Part model, mm, in its own coordinate system. A direction names the side the tool comes from. Round coordinates to 2 decimals unless told otherwise and drop trailing zeros. Write each loop counter-clockwise with the first axis right and the second up, starting at its lowest first coordinate (ties: lowest second). Pieces come first, ordered by that corner, then holes. Notation, with made-up numbers: M 18.5,31 L 42.5,31 A10 ccw 42.5,50 Z; hole C -17,41.5 d9. An arc over 180 degrees is marked long. One line per question, with ' | ' between items. Start each with the question number.
1) Saw through at C-C (x = -12.7). List the corners of the cut face in (y, z), plus the area to 3 significant figures.
2) Saw through at B-B (y = 25.4). List the corners of the cut face in (x, z), plus the area to 3 significant figures.
3) Tool access for faces 4 (the face through (-25.4, 113, 13)), 5 (the face through (-72, 239, 23.812)), 6 (the face through (-130, 252.412, 13)): list every direction of +Z, -Z, +X, -X, +Y, -Y with a clear straight run to the whole face (end or side of a thin tool).
4) Wall check: probe 1 along Y at (x, z) = (-73, 13); probe 2 along X at (y, z) = (34, 16); probe 3 along Y at (x, z) = (-12.7, 0.9). Give the ranges that are in metal, low to high. Write a range as [from, to].
5) Drop flat-ended pins along their axis: pin 1 Ø12 at (x, z) = (-178, 11.5) entering from -Y; pin 2 Ø8 at (y, z) = (185, 3.5) entering from -X. Give the stop position or say it passes through.
6) Saw through at D-D (y = 241.3). List the corners of the cut face in (x, z), plus the area to 3 significant figures.
7) Saw through at A-A (z = 9.75). List the corners of the cut face in (x, y), plus the area to 3 significant figures.
8) Mould opens along X. For faces 1 (the face through (-249.018, 242.731, 0.783)), 2 (the face through (-137, 230.188, 13)), 3 (the face through (0, 129, 13)) say: pulls with the +X half, pulls with the -X half, needs draft (parallel to the pull), parting line crosses it, or undercut.
Autodesk Inventor part; units mm, degrees
ref_plane "YZ Plane" through (0, 0, 0) normal (1, 0, 0) x (0, 1, 0)
ref_plane "XZ Plane" through (0, 0, 0) normal (0, 1, 0) x (-1, 0, 0)
ref_plane "XY Plane" through (0, 0, 0) normal (0, 0, 1) x (1, 0, 0)
sketch "Sketch1" plane through (0, 0, 0) normal (0, 0, 1) x (1, 0, 0)
  line L0 (0, 0) -> (-25.4, 0)
  line L1 (-254, 228.6) -> (-254, 254)
  line L2 (-254, 254) -> (0, 254)
  line L3 (0, 254) -> (0, 0)
  line L4 (-25.4, 0) -> (-25.4, 228.6)
  line L5 (-25.4, 228.6) -> (-254, 228.6)
  dimension "d0" = 25.4
  dimension "d1" = 254
  dimension "d2" = 254
extrude "Extrusion1" add sketch "Sketch1" along normal blind 25.4
shell "Shell1" thickness 1.5875 removed faces 2 at (-8.4667, 0, 8.4667) at (-254, 237.0667, 8.4667)
sketch "Sketch2" plane through (0, 0, 25.4) normal (0, 0, 1) x (1, 0, 0)
  line L0 (0, 0) -> (-25.4, 0)
  line L1 (0, 254) -> (0, 0)
  circle A0 centre (-12.7, 25.4) radius 4.7625
  dimension "d6" = 9.525
  dimension "d7" = 12.7
  dimension "d8" = 25.4
extrude "Extrusion2" cut sketch "Sketch2" against normal through all
sketch "Sketch3" plane through (0, 0, 0) normal (0, 0, -1) x (-1, 0, 0)
  line L0 (25.4, 228.6) -> (254, 228.6)
  line L1 (254, 228.6) -> (254, 254)
  circle A0 centre (244.475, 241.3) radius 4.7625
  dimension "d11" = 9.525
  dimension "d12" = 12.7
  dimension "d13" = 9.525
extrude "Extrusion3" cut sketch "Sketch3" against normal through all
properties part number "LoweringArm" material "Aluminum-6061"
Answer key:
1) outline: M 0,0 L 20.64,0 L 20.64,1.59 L 0,1.59 Z; M 0,23.81 L 20.64,23.81 L 20.64,25.4 L 0,25.4 Z; M 30.16,0 L 254,0 L 254,25.4 L 30.16,25.4 L 30.16,23.81 L 252.41,23.81 L 252.41,1.59 L 30.16,1.59 Z | area: 811 mm2
2) outline: M -25.4,0 L -17.46,0 L -17.46,1.59 L -23.81,1.59 L -23.81,23.81 L -17.46,23.81 L -17.46,25.4 L -25.4,25.4 Z; M -7.94,0 L 0,0 L 0,25.4 L -7.94,25.4 L -7.94,23.81 L -1.59,23.81 L -1.59,1.59 L -7.94,1.59 Z | area: 121 mm2
3) face 4: +Z, -Z, -X, -Y | face 5: none | face 6: -X
4) probe 1: y = [228.6, 230.19], [252.41, 254] | probe 2: x = [-25.4, -23.81], [-1.59, 0] | probe 3: y = [0, 20.64], [30.16, 254]
5) pin 1: stops at y = 228.6 | pin 2: stops at x = -25.4
6) outline: M -254,0 L -249.24,0 L -249.24,1.59 L -254,1.59 Z; M -254,23.81 L -249.24,23.81 L -249.24,25.4 L -254,25.4 Z; M -239.71,0 L 0,0 L 0,25.4 L -239.71,25.4 L -239.71,23.81 L -1.59,23.81 L -1.59,1.59 L -239.71,1.59 Z | area: 811 mm2
7) outline: M -254,228.6 L -25.4,228.6 L -25.4,0 L -23.81,0 L -23.81,230.19 L -254,230.19 Z; M -254,252.41 L -1.59,252.41 L -1.59,0 L 0,0 L 0,254 L -254,254 Z | area: 1,530 mm2
8) face 1: undercut | face 2: needs draft | face 3: pulls with the +X half
